```python
from build123d import *

# Parameters (mm, degrees)
F1_DEPTH = 63.5
F2_DEPTH = 25.4
F3_DEPTH = 7.9375
F0_W     = 25.108041
F0_H     = 19.05
F4_DEPTH = 25.4
F6_R     = 6.35


with BuildPart() as f1:
    # F0 (on Front) → F1 (new body, symmetric)
    with BuildSketch(Plane.XZ):
        Polygon((-41.275, -9.525), (41.275, -9.525), (41.275, 9.525), (22.225, 9.525), (-41.275, 9.525), align=None)
    extrude(amount=F1_DEPTH, both=True)

    # F0 (on Front) → F2 (join, symmetric)
    with BuildSketch(Plane.XZ):
        with BuildLine():
            Line((22.225, 9.525), (41.275, 9.525))
            Line((41.275, 9.525), (41.275, 38.1))
            ThreePointArc((41.275, 38.1), (45.92468, 49.32532), (57.15, 53.975))
            Line((57.15, 53.975), (60.616959, 53.975))
            Line((60.616959, 53.975), (60.616959, 73.025))
            Line((60.616959, 73.025), (57.15, 73.025))
            add(Edge.make_bspline(
                [(56.520232, 73.019322), (56.730123, 73.021776), (56.940047, 73.023669), (57.15, 73.025)],
                knots=[116.639514, 116.639514, 116.639514, 116.639514, 117.131254, 117.131254, 117.131254, 117.131254], degree=3))
            ThreePointArc((56.520232, 73.019322), (32.232634, 62.572035), (22.225, 38.1))
            Line((22.225, 38.1), (22.225, 9.525))
        make_face()
    extrude(amount=F2_DEPTH, both=True)

    # F0 (on Front) → F3 (join, symmetric)
    with BuildSketch(Plane.XZ):
        with BuildLine():
            add(Edge.make_bspline(
                [(-41.275, 9.525), (-41.24459, 40.322047), (6.734345, 72.437214), (56.520232, 73.019322)],
                knots=[0, 0, 0, 0, 116.639514, 116.639514, 116.639514, 116.639514], degree=3))
            Line((-41.275, 9.525), (22.225, 9.525))
            Line((22.225, 9.525), (22.225, 38.1))
            ThreePointArc((22.225, 38.1), (32.232634, 62.572035), (56.520232, 73.019322))
        make_face()
    extrude(amount=F3_DEPTH, both=True)

    # F0 (on Front) → F4 (join, symmetric)
    with BuildSketch(Plane.XZ):
        with Locations((73.170979, 63.5)):
            Rectangle(F0_W, F0_H)
    extrude(amount=F4_DEPTH, both=True)

    # F0 (on Front) → F5 (revolve)
    with BuildSketch(Plane.XZ):
        Polygon((85.725, 73.025), (85.725, 53.975), (85.725, 50.250445), (111.416959, 50.250445), (111.416959, 78.825445), (85.725, 78.825445), align=None)
    revolve(axis=Axis((85.725, 0, 64.537945), (0, 0, -1)))

    # F6
    f6_edges = [f1.edges().sort_by_distance(p)[0] for p in [
        (-41.275, -63.5, 0),
        (41.275, -63.5, 0),
        (41.275, 63.5, 0),
        (-41.275, 63.5, 0),
    ]]
    fillet(f6_edges, radius=F6_R)


solid = f1.part
```
For this review, take the finished solid that the model builds, in its own axes (mm). A direction names the side the tool comes from. Give positions to 0.01 mm unless a question says otherwise; leave off trailing zeros. Order: outer loops, then holes, each group sorted by start corner. A loop starts at its lowest first (then second) coordinate and runs counter-clockwise, first axis right, second up.
1) Take a section at B-B (y = 31). Give the boundary of the cut face in (x, z) (3 decimals), then the cut area to 3 significant figures.
2) Wall thickness on line 1 (Z direction, x = 67, y = 20) (3 decimals); line 2 (Y direction, x = 43, z = 59.5); line 3 (Y direction, x = 6.5, z = 22): over which ranges is each line inside the solid? List them lowest first.
3) Take a section at D-D (x = 92). Give the boundary of the cut face in (y, z), then the cut area to 3 significant figures.
4) Insertion check: pin 1 (14.5 mm diameter, centred on y = 13, z = 20, fed in from +X) (3 decimals); pin 2 (18 mm diameter, centred on x = 39, z = 49.5, fed in from +Y); pin 3 (5 mm diameter, centred on y = -13, z = 30.5, fed in from -X) (3 decimals); pin 4 (3 mm diameter, centred on y = -1.5, z = 60.5, fed in from +X). Each pin has a flat end and moves straight along its axis. Give the tip position at first contact, or say it passes through.
5) The part is to be moulded in two halves that separate along X. For faces 6 (the face through (59, 2, 53.975)), 7 (the face through (-39.365, -61.689, -0.133)), 8 (the face through (0, 63.5, 0)), say which applies: released by +X, released by -X, zero draft, split by the parting line, or undercut.
6) Take a section at A-A (z = -0.5). Give the boundary of the cut face in (x, y) (3 decimals), then the cut area to 3 significant figures.
7) For faces 1 (the face through (59, 0, 73.025)), 2 (the face through (85, 0, 78.825)), 3 (the face through (86, 0, 50.25)), 4 (the face through (22.225, -17, 24)), 5 (the face through (32.5, 16.55, 62.84)), list the 3-axis set-ups (+Z, -Z, +X, -X, +Y, -Y) from which the entire face can be reached by the end or side of a thin tool; tool diameter is ignored.
8) Take a section at C-C (x = 63.5). Give the boundary of the cut face in (y, z) (3 decimals).
Derived:
1. outline: (-41.275, -9.525) - (41.275, -9.525) - (41.275, 9.525) - (-41.275, 9.525) - close
1. area: 1,570 mm2
2. line 1: z = 53.975 to 73.025
2. line 2: y = -25.4 to 25.4
2. line 3: y = -7.94 to 7.94
3. outline: (-24.91, 50.25) - (24.91, 50.25) - (24.91, 78.83) - (-24.91, 78.83) - close
3. area: 1,420 mm2
4. pin 1: stops at x = 41.275
4. pin 2: stops at y = 25.4
4. pin 3: stops at x = 22.225
4. pin 4: stops at x = 111.42
5. face 6: undercut
5. face 7: released by -X
5. face 8: zero draft
6. outline: (-41.275, -57.15) arc R6.35 ccw to (-34.925, -63.5) - (34.925, -63.5) arc R6.35 ccw to (41.275, -57.15) - (41.275, 57.15) arc R6.35 ccw to (34.925, 63.5) - (-34.925, 63.5) arc R6.35 ccw to (-41.275, 57.15) - close
6. area: 10,400 mm2
7. face 1: +Z, -X
7. face 2: +Z, +X, -X, +Y, -Y
7. face 3: -Z, +X, +Y, -Y
7. face 4: +Z, -X, -Y
7. face 5: +Z, -X, +Y
8. outline: (-25.4, 53.975) - (-12.889, 53.975) - (-12.889, 50.25) - (12.889, 50.25) - (12.889, 53.975) - (25.4, 53.975) - (25.4, 73.025) - (12.889, 73.025) - (12.889, 78.825) - (-12.889, 78.825) - (-12.889, 73.025) - (-25.4, 73.025) - close
